from build123d import *

# Parameters (mm, degrees)
SKETCH_1_W          = 61.702142611
SKETCH_1_H          = 61.347239899
EXTRUDE_1_DEPTH     = 2
SKETCH_2_W          = 9
SKETCH_2_H          = 7
CUT_EXTRUDE_1_DEPTH = 2


with BuildPart() as part:
    # 草图1 → 凸台-拉伸1 (new body)
    with BuildSketch(Plane(origin=(-113.392096834, -3018.473189006, -237.947347726), x_dir=(1, 0, 0), z_dir=(0, 1, 0))):
        with BuildLine():
            Line((-117.231072015, -153.924864972), (-43.528929404, -153.924864972))
            ThreePointArc((-43.528929404, -153.924864972), (-42.114715842, -154.510651409), (-41.528929404, -155.924864972))
            Line((-41.528929404, -155.924864972), (-41.528929404, -227.272104871))
            ThreePointArc((-41.528929404, -227.272104871), (-42.114715842, -228.686318433), (-43.528929404, -229.272104871))
            Line((-43.528929404, -229.272104871), (-117.231072015, -229.272104871))
            ThreePointArc((-117.231072015, -229.272104871), (-118.645285578, -228.686318433), (-119.231072015, -227.272104871))
            Line((-119.231072015, -227.272104871), (-119.231072015, -155.924864972))
            ThreePointArc((-119.231072015, -155.924864972), (-118.645285578, -154.510651409), (-117.231072015, -153.924864972))
        make_face()
        with Locations((-80.38000071, -191.598484922)):
            Rectangle(SKETCH_1_W, SKETCH_1_H, mode=Mode.SUBTRACT)
    extrude(amount=EXTRUDE_1_DEPTH)

    # 草图2 → 切除-拉伸1 (cut)
    with BuildSketch(Plane(origin=(0, -3016.473189006, 0), x_dir=(1, 0, 0), z_dir=(0, 1, 0))):
        with Locations((-215.784101988, 80.522482755)):
            Rectangle(SKETCH_2_W, SKETCH_2_H)
    extrude(amount=-CUT_EXTRUDE_1_DEPTH, mode=Mode.SUBTRACT)


solid = part.part
Geometry: final body of the model. Coordinates: model frame, mm. A direction names the side the tool comes from. Coordinates: 2 decimals unless noted, no trailing zeros. Order: outer loops, then holes, each group sorted by start corner. A loop starts at its lowest first (then second) coordinate and runs counter-clockwise, first axis right, second up. Notation, with made-up numbers: (8, -26) - (26, -26) arc R18 cw to (26, -4) - close; hole circle Ø8 at (59, 81.25). An arc over 180 degrees is marked (long way). Use one line per item in the form item = value.
1) Section D-D (x = -216). Return loops of the section in (y, z), then the cut area to 3 significant figures.
Solutions:
outline = (-3018.47, -15.68) - (-3016.47, -15.68) - (-3016.47, -8.68) - (-3018.47, -8.68) - close
area = 14.0 mm^2
2) Set-up query: faces 5 (the face through (-187, -3017, -77.022)), 6 (the face through (-226, -3017, -84.022)), 7 (the face through (-211.284, -3017, -80)). Return all of +Z, -Z, +X, -X, +Y, -Y with unobstructed straight access to the full face (end or side cutting, diameter ignored); none if empty.
Solutions:
face_5 = +Y, -Y
face_6 = -Z, +X, -X, +Y, -Y
face_7 = -Z, +Y, -Y
3) Section A-A (x = -181.5). Return loops of the section in (y, z).
Solutions:
outline = (-3018.47, -84.02) - (-3016.47, -84.02) - (-3016.47, -77.02) - (-3018.47, -77.02) - close; (-3018.47, -15.68) - (-3016.47, -15.68) - (-3016.47, -8.68) - (-3018.47, -8.68) - close
4) Section C-C (y = -3017.45). Return loops of the section in (x, z).
Solutions:
outline = (-232.62, -82.02) arc R2 ccw to (-230.62, -84.02) - (-220.28, -84.02) - (-220.28, -77.02) - (-224.62, -77.02) - (-224.62, -15.68) - (-162.92, -15.68) - (-162.92, -77.02) - (-211.28, -77.02) - (-211.28, -84.02) - (-156.92, -84.02) arc R2 ccw to (-154.92, -82.02) - (-154.92, -10.68) arc R2 ccw to (-156.92, -8.68) - (-230.62, -8.68) arc R2 ccw to (-232.62, -10.68) - close
5) Pin query (flat end, axial travel): pin 1 (6 mm diameter, centred on x = -219, z = -57.5, fed in from -Y). Return the tip coordinate at first contact, or that it passes through.
Solutions:
pin_1 = through
6) Ray query, L1, parallel to Z at x = -195.5, y = -3017.35; L2, parallel to X at y = -3017.85, z = -51.5. Return the intervals inside material, ascending.
Solutions:
L1 = -84.02 to -77.02, -15.68 to -8.68
L2 = -232.62 to -224.62, -162.92 to -154.92
7) Mould query, pull axis X, two halves, no side actions, for faces 1 (the face through (-184, -3017, -84.022)), 2 (the face through (-155.49, -3017.49, -9.28)), 3 (the face through (-220.284, -3017, -80)), 4 (the face through (-222, -3017, -77.022)). Classes: +X half, -X half, draft (parallel to the pull), parting line (faces both ways), or undercut.
Solutions:
face_1 = draft
face_2 = +X half
face_3 = undercut
face_4 = undercut
8) Section B-B (z = -66). Return loops of the section in (x, y).
Solutions:
outline = (-232.62, -3018.47) - (-224.62, -3018.47) - (-224.62, -3016.47) - (-232.62, -3016.47) - close; (-162.92, -3018.47) - (-154.92, -3018.47) - (-154.92, -3016.47) - (-162.92, -3016.47) - close
